Check sheet for the modelled part. Datum: model origin and axes. Units: mm. A direction names the side the tool comes from. Round coordinates to 2 decimals unless told otherwise and drop trailing zeros. Loops run counter-clockwise (first coordinate to the right, second up) from the corner with the lowest first, then second, coordinate; pieces in that order, holes last. Notation, with made-up numbers: (32.25, 19.25) - (91.25, 19.25) arc R31 cw to (91.25, 55.25) - close; hole circle Ø8 at (-1.5, 46). An arc over 180 degrees is marked (long way). Put each result on its own line as item: value. Start each with the question number.
Item 1: Gauge pin test, flat ends, axial feed: pin 1 Ø11 at (y, z) = (2, -45) entering from +X; pin 2 Ø0.8 at (x, y) = (14, 4.5) entering from +Z; pin 3 Ø1.8 at (x, y) = (14.5, 4.5) entering from -Z; pin 4 Ø3 at (x, y) = (127, -39) entering from +Z. Record the tip position at first contact, or that the pin passes through.
Item 2: Draft check along Y on faces 5 (the flat face through (2, -4, -4)), 6 (the cylindrical face through (101.55, -8.02, 36.12)), 7 (the cylindrical face through (54, 0, -43)). Enter one of: pulls with the +Y half, pulls with the -Y half, needs draft (parallel to the pull), parting line crosses it, or undercut.
Item 3: Section check A-A, the plane y = -46. Record the cut outline in (x, z), and give its area (3 significant figures).
Item 4: Tool access check on faces 1 (the flat face through (3, 4, -4)), 2 (the cylindrical face through (51.014, 23.846, -7.509)), 3 (the cylindrical face through (54, -43, 0)), 4 (the cylindrical face through (59.465, -41.043, 0.651)). Record the directions out of +Z, -Z, +X, -X, +Y, -Y that give a thin tool (end or side, any length) a straight path to the whole face; none if there is none.
Item 5: Section check C-C, the plane z = 0. Give the number of separate pieces and of enclosed holes in the cut face, and give its area (3 significant figures).
Item 6: Material ranges on line 1 along Z through (x, y) = (55.15, 0); line 2 along Y through (x, z) = (59.8, 0), recorded low to high.
from build123d import *

# Parameters (mm, degrees)
R_P_TITION_CIRCULAIRE1_COUNT = 4
ENL_V_MAT_EXTRU_1_DEPTH      = 10


with BuildPart() as part:
    # Esquisse1 → Révolution1 (revolve)
    with BuildSketch(Plane.XY):
        Polygon((0, 0), (0, 5), (1, 6), (2, 6), (2, 5), (3, 5), (3, 6), (30, 6), (30, 10), (49, 10), (49, 24), (50, 25), (52, 25), (52, 55), (62, 55), (62, 37), (140, 37), (142, 35), (142, 0), align=None)
    revolve(axis=Axis((142, 0, 0), (-1, 0, 0)))

    # Esquisse2 → Enlèvement de matière-Révolution1 (revolve, cut)
    with BuildSketch(Plane.XY, mode=Mode.PRIVATE) as enl_vement_de_mati_re_r_volution1_sk:
        Polygon((44.05702844, 46), (69.730898062, 46), (69.730898062, 51), (57, 51), (57, 49), (44.05702844, 49), align=None)
    enl_vement_de_mati_re_r_volution1 = revolve(enl_vement_de_mati_re_r_volution1_sk.sketch.rotate(Axis((44.05702844, 46, 0), (1, 0, 0)), 90), axis=Axis((44.05702844, 46, 0), (1, 0, 0)), mode=Mode.SUBTRACT)  # turned: the seam where the file's is

    # Répétition circulaire1: Enlèvement de matière-Révolution1 ×4 about axis
    r_p_tition_circulaire1_axis = Axis((0, 0, 0), (1, 0, 0))
    for i in range(1, R_P_TITION_CIRCULAIRE1_COUNT):
        add(enl_vement_de_mati_re_r_volution1.rotate(r_p_tition_circulaire1_axis, i * 360 / R_P_TITION_CIRCULAIRE1_COUNT), mode=Mode.SUBTRACT)

    # Esquisse3 → Enlèv. mat.-Extru.1 (cut)
    with BuildSketch(Plane(origin=(0, 4, 0), x_dir=(1, 0, 0), z_dir=(0, 1, 0))):
        with BuildLine():
            Line((7, 2), (19, 2))
            ThreePointArc((19, 2), (21, 0), (19, -2))
            Line((19, -2), (7, -2))
            ThreePointArc((7, -2), (5, 0), (7, 2))
        make_face()
    extrude(amount=ENL_V_MAT_EXTRU_1_DEPTH, mode=Mode.SUBTRACT)


solid = part.part
Check result:
1. pin 1: x = 62
1. pin 2: z = 4.38
1. pin 3: z = -4.8
1. pin 4: through
2. face 5: needs draft
2. face 6: parting line crosses it
2. face 7: undercut
3. outline: (52, -30.15) - (62, -30.15) - (62, -5) - (57, -5) - (57, -3) - (52, -3) - close; (52, 3) - (57, 3) - (57, 5) - (62, 5) - (62, 30.15) - (52, 30.15) - close
3. area: 523 mm²
4. face 1: none
4. face 2: -X
4. face 3: +X, -X
4. face 4: +X
5. separate pieces: 3
5. enclosed holes: 0
5. area: 7,710 mm²
6. line 1: -55 to -49, -43 to 43, 49 to 55
6. line 2: -55 to -51, -41 to 41, 51 to 55
